```python
from build123d import *

# Parameters (mm, degrees)
BASE_EXTRUDE_DEPTH  = 8.636
SHELL1_T            = -1.1176
SKETCH2_R           = 32.131
BOSS_EXTRUDE1_DEPTH = 13.6144
SKETCH3_R           = 32.2326
BOSS_EXTRUDE2_DEPTH = 1.5748
CUT_EXTRUDE2_START  = -1.5748
CUT_EXTRUDE2_DEPTH  = 1.5748
SKETCH5_R           = 29.972
CUT_EXTRUDE3_DEPTH  = 15.367
SKETCH6_R           = 20.5105
CUT_EXTRUDE4_DEPTH  = 7.8834
CUT_EXTRUDE5_DEPTH  = 7.8834
CIRPATTERN1_COUNT   = 4
CUT_EXTRUDE6_DEPTH  = 14.224
CUT_EXTRUDE7_DEPTH  = 14.224
CUT_EXTRUDE8_DEPTH  = 14.224
CIRPATTERN2_COUNT   = 2
CIRPATTERN2_ANGLE   = 310
FILLET1_R           = 1.27


with BuildPart() as part:
    # Sketch1 → Base-Extrude (new body)
    with BuildSketch(Plane.XY):
        with BuildLine():
            Line((3.81, 0), (63.246, 0))
            ThreePointArc((63.246, 0), (65.940076836, 1.115923164), (67.056, 3.81))
            Line((67.056, 3.81), (67.056, 63.246))
            ThreePointArc((67.056, 63.246), (65.940076836, 65.940076836), (63.246, 67.056))
            Line((63.246, 67.056), (3.81, 67.056))
            ThreePointArc((3.81, 67.056), (1.115923164, 65.940076836), (0, 63.246))
            Line((0, 63.246), (0, 3.81))
            ThreePointArc((0, 3.81), (1.115923164, 1.115923164), (3.81, 0))
        make_face()
    extrude(amount=-BASE_EXTRUDE_DEPTH)

    # Shell1
    shell1_openings = [part.faces().sort_by_distance(p)[0] for p in [
        (33.528, 33.528, -8.636),
    ]]
    offset(amount=SHELL1_T, openings=shell1_openings, kind=Kind.INTERSECTION)

    # Sketch2 → Boss-Extrude1 (add)
    with BuildSketch(Plane.XY):
        with Locations((33.528, 33.528)):
            Circle(SKETCH2_R)
    extrude(amount=BOSS_EXTRUDE1_DEPTH)

    # Sketch3 → Boss-Extrude2 (add)
    with BuildSketch(Plane(origin=(0, 0, -1.1176), x_dir=(-1, 0, 0), z_dir=(0, 0, -1))):
        with Locations((-33.528, 33.528)):
            Circle(SKETCH3_R)
    extrude(amount=BOSS_EXTRUDE2_DEPTH)

    # Sketch4 → Cut-Extrude2 (cut)
    with BuildSketch(Plane(origin=(0, 0, -2.6924), x_dir=(-1, 0, 0), z_dir=(0, 0, -1)).offset(CUT_EXTRUDE2_START)):
        with BuildLine():
            Line((-63.246, 65.9384), (-3.81, 65.9384))
            ThreePointArc((-3.81, 65.9384), (-1.906185702, 65.149814298), (-1.1176, 63.246))
            Line((-1.1176, 63.246), (-1.1176, 3.81))
            ThreePointArc((-1.1176, 3.81), (-1.906185702, 1.906185702), (-3.81, 1.1176))
            Line((-3.81, 1.1176), (-63.246, 1.1176))
            ThreePointArc((-63.246, 1.1176), (-65.149814298, 1.906185702), (-65.9384, 3.81))
            Line((-65.9384, 3.81), (-65.9384, 63.246))
            ThreePointArc((-65.9384, 63.246), (-65.149814298, 65.149814298), (-63.246, 65.9384))
        make_face()
        with BuildLine():
            Line((-3.81, 63.9572), (-63.246, 63.9572))
            ThreePointArc((-63.246, 63.9572), (-63.748894343, 63.748894343), (-63.9572, 63.246))
            Line((-63.9572, 63.246), (-63.9572, 3.81))
            ThreePointArc((-63.9572, 3.81), (-63.748894343, 3.307105657), (-63.246, 3.0988))
            Line((-63.246, 3.0988), (-3.81, 3.0988))
            ThreePointArc((-3.81, 3.0988), (-3.307105657, 3.307105657), (-3.0988, 3.81))
            Line((-3.0988, 3.81), (-3.0988, 63.246))
            ThreePointArc((-3.0988, 63.246), (-3.307105657, 63.748894343), (-3.81, 63.9572))
        make_face(mode=Mode.SUBTRACT)
    extrude(amount=CUT_EXTRUDE2_DEPTH, mode=Mode.SUBTRACT)

    # Sketch5 → Cut-Extrude3 (cut)
    with BuildSketch(Plane.XY.offset(13.6144)):
        with Locations((33.528, 33.528)):
            Circle(SKETCH5_R)
    extrude(amount=-CUT_EXTRUDE3_DEPTH, mode=Mode.SUBTRACT)

    # Sketch6 → Cut-Extrude4 (cut, through all)
    with BuildSketch(Plane.XY.offset(-1.7526)):
        with Locations((33.528, 33.528)):
            Circle(SKETCH6_R)
    extrude(amount=-CUT_EXTRUDE4_DEPTH, mode=Mode.SUBTRACT)

    # Sketch7 → Cut-Extrude5 (cut, through all)
    with BuildSketch(Plane.XY.offset(-1.7526)):
        with BuildLine():
            Line((30.988, 63.392178944), (30.988, 58.481560993))
            ThreePointArc((30.988, 58.481560993), (38.783174993, 58.053801558), (46.06925, 55.25008219))
            Line((46.06925, 55.25008219), (48.514, 59.484513402))
            ThreePointArc((48.514, 59.484513402), (40.050514201, 62.781676564), (30.988, 63.392178944))
        make_face()
    cut_extrude5 = extrude(amount=-CUT_EXTRUDE5_DEPTH, mode=Mode.SUBTRACT)

    # CirPattern1: Cut-Extrude5 ×4 about axis
    cirpattern1_axis = Axis((33.528, 33.528, 0), (0, 0, 1))
    for i in range(1, CIRPATTERN1_COUNT):
        add(cut_extrude5.rotate(cirpattern1_axis, i * 360 / CIRPATTERN1_COUNT), mode=Mode.SUBTRACT)

    # Sketch8 → Cut-Extrude6 (cut)
    with BuildSketch(Plane(origin=(0, 0, -2.6924), x_dir=(-1, 0, 0), z_dir=(0, 0, -1))):
        with BuildLine():
            Line((-45.972542384, 63.261379687), (-44.832330284, 61.286474397))
            ThreePointArc((-44.832330284, 61.286474397), (-48.514, 59.484513402), (-51.915378856, 57.197074397))
            Line((-51.915378856, 57.197074397), (-53.055590957, 59.171979687))
            ThreePointArc((-53.055590957, 59.171979687), (-49.6443, 61.44225043), (-45.972542384, 63.261379687))
        make_face()
    extrude(amount=-CUT_EXTRUDE6_DEPTH, mode=Mode.SUBTRACT)

    # Sketch9 → Cut-Extrude7 (cut)
    with BuildSketch(Plane(origin=(0, 0, -2.6924), x_dir=(-1, 0, 0), z_dir=(0, 0, -1))):
        with BuildLine():
            Line((-8.028645234, 53.244069824), (-9.641148651, 51.631566407))
            ThreePointArc((-9.641148651, 51.631566407), (-12.334595554, 54.721404446), (-15.424433593, 57.414851349))
            Line((-15.424433593, 57.414851349), (-13.811930176, 59.027354766))
            ThreePointArc((-13.811930176, 59.027354766), (-10.736109965, 56.319890035), (-8.028645234, 53.244069824))
        make_face()
    extrude(amount=-CUT_EXTRUDE7_DEPTH, mode=Mode.SUBTRACT)

    # Sketch10 → Cut-Extrude8 (cut)
    with BuildSketch(Plane(origin=(0, 0, -2.6924), x_dir=(-1, 0, 0), z_dir=(0, 0, -1))):
        with BuildLine():
            Line((-17.273486431, 8.346427916), (-16.309737519, 6.279661704))
            ThreePointArc((-16.309737519, 6.279661704), (-19.513159966, 4.501722912), (-22.897652399, 3.0988))
            Line((-22.897652399, 3.0988), (-23.85078467, 3.0988))
            Line((-23.85078467, 3.0988), (-24.68599656, 4.889917677))
            ThreePointArc((-24.68599656, 4.889917677), (-20.861285459, 6.364143007), (-17.273486431, 8.346427916))
        make_face()
    cut_extrude8 = extrude(amount=-CUT_EXTRUDE8_DEPTH, mode=Mode.SUBTRACT)

    # CirPattern2: Cut-Extrude8 ×2 about axis
    cirpattern2_axis = Axis((33.528, 33.528, 0), (0, 0, -1))
    for i in range(1, CIRPATTERN2_COUNT):
        add(cut_extrude8.rotate(cirpattern2_axis, i * CIRPATTERN2_ANGLE / (CIRPATTERN2_COUNT - 1)), mode=Mode.SUBTRACT)

    # Fillet1
    fillet1_edges = [part.edges().sort_by_distance(p)[0] for p in [
        (33.528, 0, 0),
        (1.115923164, 1.115923164, 0),
        (0, 33.528, 0),
        (1.115923164, 65.940076836, 0),
        (33.528, 67.056, 0),
        (65.940076836, 65.940076836, 0),
        (67.056, 33.528, 0),
        (65.940076836, 1.115923164, 0),
    ]]
    fillet(fillet1_edges, radius=FILLET1_R)


solid = part.part
```
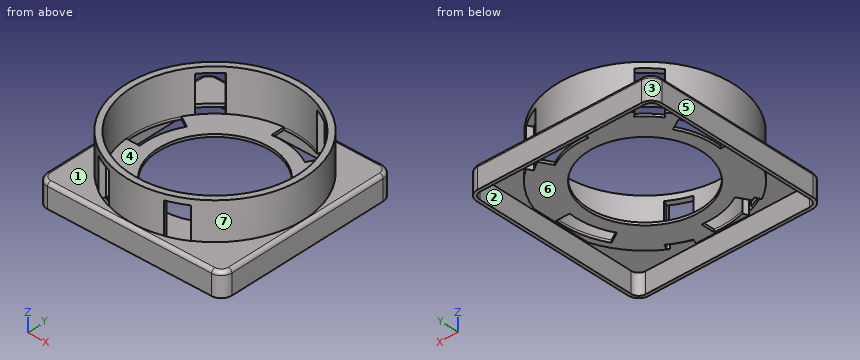
For this review, take the finished solid that the model builds, in its own axes (mm). Face numbers are marked on the shaded views. A direction names the side the tool comes from. Round coordinates to 2 decimals unless told otherwise and drop trailing zeros. Loops run counter-clockwise (first coordinate to the right, second up) from the corner with the lowest first, then second, coordinate; pieces in that order, holes last.
Q1. Add section C-C on z = 9.5. Write out the cut boundary in (x, y), plus the area to 3 significant figures.
Result sheet:
outline: (8.1, 53.17) arc R32.13 ccw to (16.35, 6.37) - (17.27, 8.35) arc R29.97 cw to (9.64, 51.63) - close; (13.88, 58.95) - (15.42, 57.41) arc R29.97 cw to (44.83, 61.29) - (45.92, 63.17) arc R32.13 ccw to start; (23.21, 3.1) arc R32.13 ccw to (43.29, 2.92) - (42.37, 4.89) arc R29.97 cw to (24.69, 4.89) - (23.85, 3.1) - close; (49.78, 8.35) - (50.62, 6.56) - (50.21, 6.06) arc R32.13 ccw to (53, 59.08) - (51.92, 57.2) arc R29.97 cw to start
area: 351 mm2
Q2. Add section A-A on x = 61. Write out the cut boundary in (y, z).
Result sheet:
outline: (0, -8.64) - (1.12, -8.64) - (1.12, -1.12) - (16.67, -1.12) - (16.67, -2.69) - (21.54, -2.69) - (21.54, 13.61) - (16.86, 13.61) - (16.86, 0) - (1.27, 0) arc R1.27 ccw to (0, -1.27) - close; (36.07, -2.69) - (50.39, -2.69) - (50.39, -1.12) - (65.94, -1.12) - (65.94, -8.64) - (67.06, -8.64) - (67.06, -1.27) arc R1.27 ccw to (65.79, 0) - (50.19, 0) - (50.19, 13.61) - (45.51, 13.61) - (45.51, -1.75) - (36.07, -1.75) - close
Q3. Add section B-B on y = 47. Write out the cut boundary in (x, z), plus the area to 3 significant figures.
Result sheet:
outline: (0, -8.64) - (1.12, -8.64) - (1.12, -1.12) - (4.25, -1.12) - (4.25, -2.69) - (6.75, -2.69) - (6.75, 13.61) - (4.36, 13.61) - (4.36, 0) - (1.27, 0) arc R1.27 ccw to (0, -1.27) - close; (10.19, -2.69) - (18.06, -2.69) - (18.06, -1.75) - (10.19, -1.75) - close; (48.99, -2.69) - (62.81, -2.69) - (62.81, -1.12) - (65.94, -1.12) - (65.94, -8.64) - (67.06, -8.64) - (67.06, -1.27) arc R1.27 ccw to (65.79, 0) - (62.7, 0) - (62.7, 13.61) - (60.3, 13.61) - (60.3, -1.75) - (48.99, -1.75) - close
area: 122 mm2
Q4. Add section D-D on x = 11. Write out the cut boundary in (y, z).
Result sheet:
outline: (0, -8.64) - (1.12, -8.64) - (1.12, -1.12) - (10.48, -1.12) - (10.48, -2.69) - (44.56, -2.69) - (44.56, -1.75) - (13.76, -1.75) - (13.76, 13.61) - (10.62, 13.61) - (10.62, 0) - (1.27, 0) arc R1.27 ccw to (0, -1.27) - close; (46.53, -2.69) - (53.3, -2.69) - (53.3, -1.75) - (46.53, -1.75) - close; (53.3, 11.53) - (56.44, 11.53) - (56.44, 13.61) - (53.3, 13.61) - close; (56.58, -1.12) - (65.94, -1.12) - (65.94, -8.64) - (67.06, -8.64) - (67.06, -1.27) arc R1.27 ccw to (65.79, 0) - (56.58, 0) - close
Q5. Insertion check: pin 1 Ø4 at (y, z) = (42, 6) entering from +X; pin 2 Ø12 at (x, z) = (7, 11) entering from +Y; pin 3 Ø8 at (x, y) = (49, 44.5) entering from +Z. Each pin has a flat end and moves straight along its axis. Give the tip position at first contact, or say it passes through.
Result sheet:
pin 1: stops at x = 65
pin 2: stops at y = 58.23
pin 3: stops at z = -1.75
Q6. Machinability: for the marked faces 1, 2 and 3, which of the approach directions +Z, -Z, +X, -X, +Y, -Y give a long, thin tool a straight path to every point of the face, cutting with its end or side? Answer none if there is none.
Result sheet:
face 1: +Z
face 2: -Z
face 3: +Z, -Z, -X, +Y
Q7. Mouldability with a two-part tool opening along Y and no side actions: class the marked faces 4, 5, 6 and 7 as +Y half, -Y half, draft (parallel to the pull), parting line (faces both ways), or undercut.
Result sheet:
face 4: undercut
face 5: draft
face 6: undercut
face 7: parting line
Q8. To check wall thickness, follow line 1 along Y through (x, z) = (54, -6.25); line 2 along Y through (x, z) = (34, 6). State the ranges of each line that lie inside material, in increasing order.
Result sheet:
line 1: y = 0 to 1.12, 65.94 to 67.06
line 2: y = 1.4 to 3.56, 63.5 to 65.66
